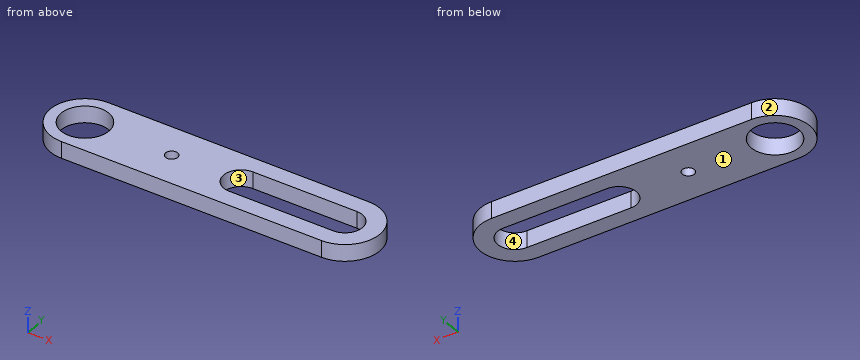
from build123d import *

# Parameters (mm, degrees)
F0_R     = 3.4925
F0_R_2   = 0.889
F1_DEPTH = 2.4384


with BuildPart() as f1:
    # F0 (on Top) → F1 (new body)
    with BuildSketch(Plane.XY):
        with BuildLine():
            Line((-38.1, -5.08), (0, -5.08))
            ThreePointArc((0, -5.08), (5.08, 0), (0, 5.08))
            Line((0, 5.08), (-38.1, 5.08))
            ThreePointArc((-38.1, 5.08), (-43.18, 0), (-38.1, -5.08))
        make_face()
        with Locations((-38.1, 0)):
            Circle(F0_R, mode=Mode.SUBTRACT)
        with Locations((-25.4, 0)):
            Circle(F0_R_2, mode=Mode.SUBTRACT)
        with BuildLine():
            ThreePointArc((0, 2.54), (2.54, 0), (0, -2.54))
            Line((0, -2.54), (-15.24, -2.54))
            ThreePointArc((-15.24, -2.54), (-17.78, 0), (-15.24, 2.54))
            Line((-15.24, 2.54), (0, 2.54))
        make_face(mode=Mode.SUBTRACT)
    extrude(amount=F1_DEPTH)


solid = f1.part
Check sheet for the modelled part. Datum: model origin and axes. Units: mm. Face numbers are marked on the shaded views. Round coordinates to 2 decimals unless told otherwise and drop trailing zeros. Order: outer loops, then holes, each group sorted by start corner. A loop starts at its lowest first (then second) coordinate and runs counter-clockwise, first axis right, second up.
(1) Cross-section at A-A, the plane x = -9.5. Enter the section's corners in (y, z).
(2) Draft check along Y on the marked faces 1, 2, 3 and 4. Enter one of: pulls with the +Y half, pulls with the -Y half, needs draft (parallel to the pull), parting line crosses it, or undercut.
(3) Cross-section at B-B, the plane z = 1.15. Enter the section's corners in (x, y) (1 decimal).
(4) Scan lines: probe 1 along Y at (x, z) = (-38.1, 1.05); probe 2 along X at (y, z) = (2.25, 1); probe 3 along X at (y, z) = (0.25, 1.45). Record each from-to range of solid material in increasing order.
(5) Cross-section at C-C, the plane y = 3. Enter the section's corners in (x, z).
(6) Cross-section at D-D, the plane y = -2. Enter the section's corners in (x, z), and give its area (3 significant figures).
(7) Go/stop test with a flat-tipped pin: P1, Ø1.4, axis at x = -25.4, y = 0, coming from the -Z side. Record where the tip stops, or that it passes through.
Check sheet entries:
1. outline: (-5.08, 0) - (-2.54, 0) - (-2.54, 2.44) - (-5.08, 2.44) - close; (2.54, 0) - (5.08, 0) - (5.08, 2.44) - (2.54, 2.44) - close
2. face 1: needs draft
2. face 2: parting line crosses it
2. face 3: undercut
2. face 4: undercut
3. outline: (-38.1, -5.1) - (0, -5.1) arc R5.1 ccw to (0, 5.1) - (-38.1, 5.1) arc R5.1 ccw to start; hole circle Ø7 at (-38.1, 0); hole circle Ø1.8 at (-25.4, 0); hole (-15.2, -2.5) - (0, -2.5) arc R2.5 ccw to (0, 2.5) - (-15.2, 2.5) arc R2.5 ccw to start
4. probe 1: y = -5.08 to -3.49, 3.49 to 5.08
4. probe 2: x = -42.65 to -40.77, -35.43 to -16.42, 1.18 to 4.55
4. probe 3: x = -43.17 to -41.58, -34.62 to -26.25, -24.55 to -17.77, 2.53 to 5.07
5. outline: (-42.2, 0) - (-39.89, 0) - (-39.89, 2.44) - (-42.2, 2.44) - close; (-36.31, 0) - (4.1, 0) - (4.1, 2.44) - (-36.31, 2.44) - close
6. outline: (-42.77, 0) - (-40.96, 0) - (-40.96, 2.44) - (-42.77, 2.44) - close; (-35.24, 0) - (-16.81, 0) - (-16.81, 2.44) - (-35.24, 2.44) - close; (1.57, 0) - (4.67, 0) - (4.67, 2.44) - (1.57, 2.44) - close
6. area: 56.9 mm2
7. P1: passes through
